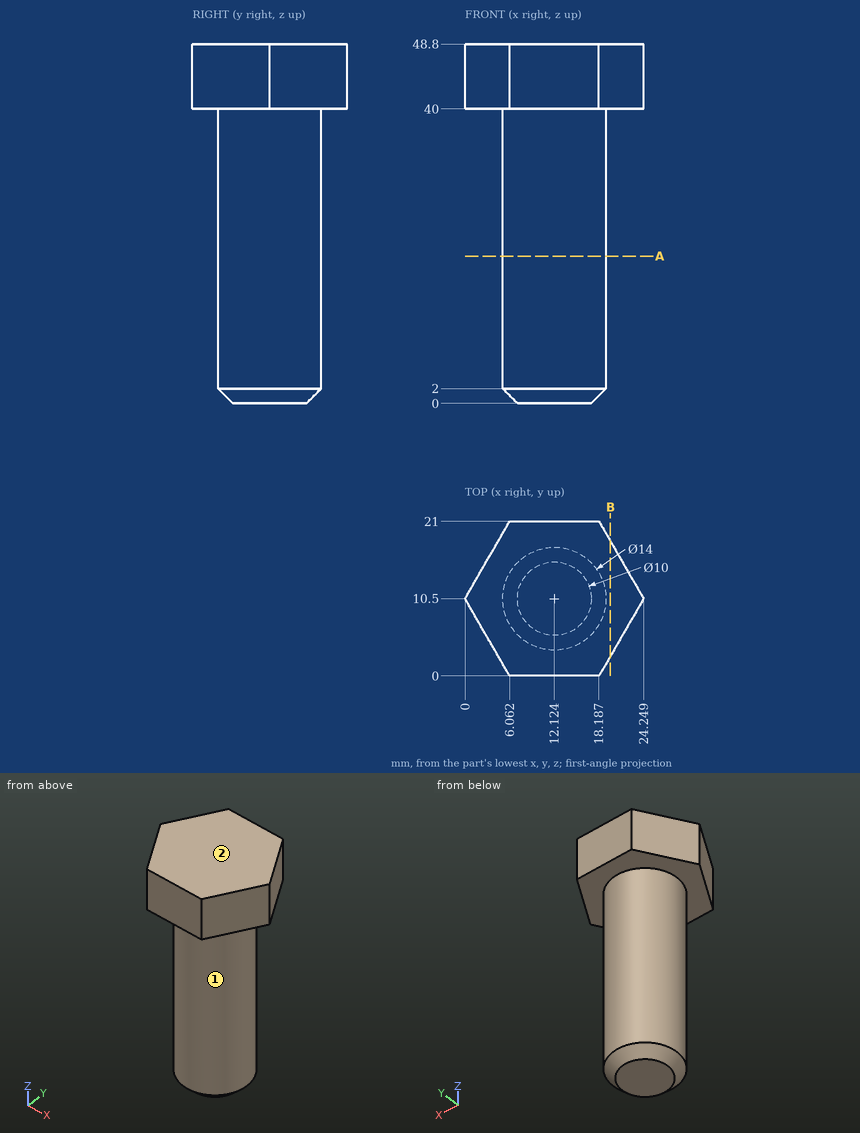
Drawing for the job (mm, zero at the part's lowest x, y, z). A direction names the side the tool comes from. Round coordinates to 2 decimals unless told otherwise and drop trailing zeros. Loops run counter-clockwise (first coordinate to the right, second up) from the corner with the lowest first, then second, coordinate; pieces in that order, holes last. Notation, with made-up numbers: (81.25, -39.75) - (96.25, -39.75) arc R17 cw to (96.25, -6.75) - close; hole circle Ø6 at (72.25, 12.25). An arc over 180 degrees is marked (long way). Return JSON: item names as keys, results as strings. Group by question number.
Q1. Drill centre lines: line 1 along Z through (x, y) = (4.5, 6.5); line 2 along X through (y, z) = (10.25, 39); line 3 along X through (y, z) = (9.75, 18) (1 decimal). Where is each one in solid material? Low to high. Write a range as [from, to].
Q2. Tool access for the marked faces 1 and 2: list every direction of +Z, -Z, +X, -X, +Y, -Y with a clear straight run to the whole face (end or side of a thin tool).
Q3. Band-saw the part on B-B on x = 19.75. Give the cut face in (y, z).
Q4. Flat gauge pins, fed straight in: pin 1 Ø2 at (x, z) = (11, 10.5) entering from -Y; pin 2 Ø6 at (x, z) = (6, 23) entering from +Y (1 decimal); pin 3 Ø5 at (x, y) = (10, 3) entering from -Z (1 decimal). Where does each tip first touch, or does it go through?
Q5. Band-saw the part on A-A on z = 20. Give the cut face in (x, y) (1 decimal).
Solutions:
{
 "1": {"line 1": "z = [40, 48.8]", "line 2": "x = [5.13, 19.12]", "line 3": "x = [5.2, 19.1]"},
 "2": {"face 1": "-Z", "face 2": "+Z, +X, -X, +Y, -Y"},
 "3": {"outline": "(2.71, 40) - (18.29, 40) - (18.29, 48.8) - (2.71, 48.8) - close"},
 "4": {"pin 1": "stops at y = 3.5", "pin 2": "stops at y = 16.8", "pin 3": "stops at z = 0.3"},
 "5": {"outline": "circle Ø14 at (12.1, 10.5)"}
}
